```python
from build123d import *

# Parameters (mm, degrees)
F0_R     = 5.3351790251
F1_DEPTH = 10
F2_DEPTH = 10
F3_COUNT = 14
F4_R     = 15.5
F5_DEPTH = 10
F8_DEPTH = 10
F7_R     = 2
F9_DEPTH = 10


# Not quite as in the source:
# - a feature names something its author has since deleted; it is built from what else it names


with BuildPart() as f1:
    # F0 (on Top) → F1 (new body)
    with BuildSketch(Plane.XY):
        Circle(F0_R)
    extrude(amount=F1_DEPTH)



with BuildPart() as f2:
    # F0 (on Top) → F2 (new body)
    with BuildSketch(Plane.XY):
        with BuildLine():
            Line((-21.0813645951, 0), (-15.5169374102, 0))
            Line((-15.5169374102, 0), (-15.5169374102, 2.1929510403))
            add(Edge.make_bspline(
                [(-15.5169374102, 2.1929510403), (-15.7431787684, 2.1963284468), (-16.4584927159, 2.2070069607), (-21.1021855068, 0.9410331304), (-21.0859014535, 0.2050513008), (-21.0813645951, 0)],
                knots=[0, 0, 0, 0, 0.2502118821, 0.7911020914, 1, 1, 1, 1], degree=3))
        make_face()
        Polygon((-15.5169374102, -2.1929510403), (-13.8607590251, -2.1929510403), (-13.8607590251, 2.1929510403), (-15.5169374102, 2.1929510403), (-15.5169374102, 0), align=None)
        with BuildLine():
            add(Edge.make_bspline(
                [(-15.5169374102, -2.1929510403), (-15.7431787684, -2.1963284468), (-16.4584927159, -2.2070069607), (-21.1021855068, -0.9410331304), (-21.0859014535, -0.2050513008), (-21.0813645951, 0)],
                knots=[0, 0, 0, 0, 0.2502118821, 0.7911020914, 1, 1, 1, 1], degree=3))
            Line((-15.5169374102, -2.1929510403), (-15.5169374102, 0))
            Line((-15.5169374102, 0), (-21.0813645951, 0))
        make_face()
    extrude(amount=F2_DEPTH)


with BuildPart() as f3_1:
    # F3: instance of F2
    add(f2.part.rotate(Axis((0, 0, 10), (0, 0, 1)), 1 * 360 / F3_COUNT))


with BuildPart() as f3_2:
    # F3: instance of F2
    add(f2.part.rotate(Axis((0, 0, 10), (0, 0, 1)), 2 * 360 / F3_COUNT))


with BuildPart() as f3_3:
    # F3: instance of F2
    add(f2.part.rotate(Axis((0, 0, 10), (0, 0, 1)), 3 * 360 / F3_COUNT))


with BuildPart() as f3_4:
    # F3: instance of F2
    add(f2.part.rotate(Axis((0, 0, 10), (0, 0, 1)), 4 * 360 / F3_COUNT))


with BuildPart() as f3_5:
    # F3: instance of F2
    add(f2.part.rotate(Axis((0, 0, 10), (0, 0, 1)), 5 * 360 / F3_COUNT))


with BuildPart() as f3_6:
    # F3: instance of F2
    add(f2.part.rotate(Axis((0, 0, 10), (0, 0, 1)), 6 * 360 / F3_COUNT))


with BuildPart() as f3_7:
    # F3: instance of F2
    add(f2.part.rotate(Axis((0, 0, 10), (0, 0, 1)), 7 * 360 / F3_COUNT))


with BuildPart() as f3_8:
    # F3: instance of F2
    add(f2.part.rotate(Axis((0, 0, 10), (0, 0, 1)), 8 * 360 / F3_COUNT))


with BuildPart() as f3_9:
    # F3: instance of F2
    add(f2.part.rotate(Axis((0, 0, 10), (0, 0, 1)), 9 * 360 / F3_COUNT))


with BuildPart() as f3_10:
    # F3: instance of F2
    add(f2.part.rotate(Axis((0, 0, 10), (0, 0, 1)), 10 * 360 / F3_COUNT))


with BuildPart() as f3_11:
    # F3: instance of F2
    add(f2.part.rotate(Axis((0, 0, 10), (0, 0, 1)), 11 * 360 / F3_COUNT))


with BuildPart() as f3_12:
    # F3: instance of F2
    add(f2.part.rotate(Axis((0, 0, 10), (0, 0, 1)), 12 * 360 / F3_COUNT))


with BuildPart() as f3_13:
    # F3: instance of F2
    add(f2.part.rotate(Axis((0, 0, 10), (0, 0, 1)), 13 * 360 / F3_COUNT))


with BuildPart() as f1_1:
    add(f1.part)

    add(f2.part)  # F5 merges F2

    add(f3_1.part)  # F5 merges F3_1

    add(f3_2.part)  # F5 merges F3_2

    add(f3_3.part)  # F5 merges F3_3

    add(f3_4.part)  # F5 merges F3_4

    add(f3_5.part)  # F5 merges F3_5

    add(f3_6.part)  # F5 merges F3_6

    add(f3_7.part)  # F5 merges F3_7

    add(f3_8.part)  # F5 merges F3_8

    add(f3_9.part)  # F5 merges F3_9

    add(f3_10.part)  # F5 merges F3_10

    add(f3_11.part)  # F5 merges F3_11

    add(f3_12.part)  # F5 merges F3_12

    add(f3_13.part)  # F5 merges F3_13
    # F4 (on Top) → F5 (join)
    with BuildSketch(Plane.XY):
        Circle(F4_R)
    extrude(amount=F5_DEPTH)

    # F6 (on face) → F8 (cut, through all)
    with BuildSketch(Plane.XY.offset(10)):
        with BuildLine():
            ThreePointArc((-5.9088465181, -1.041889066), (-5.1961524227, 3), (-2.05212086, 5.6381557247))
            Line((-2.05212086, 5.6381557247), (-4.1564424219, 11.4197316993))
            ThreePointArc((-4.1564424219, 11.4197316993), (-10.5244816627, 6.076312321), (-11.967998967, -2.110281123))
            Line((-11.967998967, -2.110281123), (-5.9088465181, -1.041889066))
        make_face()
        with BuildLine():
            Line((-3.8567256581, -4.5962666587), (-7.8115565451, -9.3094505764))
            ThreePointArc((-7.8115565451, -9.3094505764), (0, -12.1526246421), (7.8115565451, -9.3094505764))
            Line((7.8115565451, -9.3094505764), (3.8567256581, -4.5962666587))
            ThreePointArc((3.8567256581, -4.5962666587), (0, -6), (-3.8567256581, -4.5962666587))
        make_face()
        with BuildLine():
            ThreePointArc((2.05212086, 5.6381557247), (5.1961524227, 3), (5.9088465181, -1.041889066))
            Line((5.9088465181, -1.041889066), (11.967998967, -2.110281123))
            ThreePointArc((11.967998967, -2.110281123), (10.5244816627, 6.076312321), (4.1564424219, 11.4197316993))
            Line((4.1564424219, 11.4197316993), (2.05212086, 5.6381557247))
        make_face()
    extrude(amount=-F8_DEPTH, mode=Mode.SUBTRACT)

    # F7 (on face) → F9 (cut, through all)
    with BuildSketch(Plane.XY.offset(10)):
        Circle(F7_R)
    extrude(amount=-F9_DEPTH, mode=Mode.SUBTRACT)


solid = f1_1.part
```
Source: CAD feature listing. Evaluate the final solid. Frame: model axes, mm. A direction names the side the tool comes from. Round coordinates to 2 decimals unless told otherwise and drop trailing zeros. Write each loop counter-clockwise with the first axis right and the second up, starting at its lowest first coordinate (ties: lowest second). Pieces come first, ordered by that corner, then holes. Notation, with made-up numbers: M -24.5,7 L 7.5,7 A24 ccw 7.5,22 Z; hole C -27,85.25 d8. An arc over 180 degrees is marked long. Answer as a JSON object with one key per item and string values. Group by question number.
(1) Section query A-A on x = 0. Output: boundary loops of the cut face in (y, z).
(2) Section query C-C on z = 5.25. State how many separate pieces and enclosed holes the cut face has, then the cut area to 3 significant figures.
(3) Ray query, line 1 (Y direction, x = 0, z = 7.75); line 2 (X direction, y = 7.5, z = 9.25); line 3 (Y direction, x = -17, z = 1.5). Return the intervals inside material, ascending. Write a range as [from, to].
(4) Section query B-B on x = -7. Output: boundary loops of the cut face in (y, z).
(5) Mould query, pull axis X, two halves, no side actions, for faces 1 (the cylindrical face through (15.1, -3.5, 4.9)), 2 (the flat face through (0, 4, 0)), 3 (the cylindrical face through (12.107, -9.678, 4.93)). Classes: +X half, -X half, draft (parallel to the pull), parting line (faces both ways), or undercut.
(6) First-contact query: pin 1 (3 mm diameter, centred on y = 15.5, z = 7.5, fed in from +X); pin 2 (1.5 mm diameter, centred on y = 14, z = 5, fed in from +X). Flat tips, straight axial feed; report the tip coordinate or a pass-through.
(7) Reachability of faces 4 (the cylindrical face through (5.167, 3.051, 5.07)), 5 (the flat face through (0, 4, 10)), 6 (the cylindrical face through (-15.1, 3.5, 4.9)) from +Z, -Z, +X, -X, +Y, -Y: full face, straight path, thin tool, end or side. Return the list, or none.
Computed values:
{
 "1": {"outline": "M -15.5,0 L -12.15,0 L -12.15,10 L -15.5,10 Z; M -6,0 L -2,0 L -2,10 L -6,10 Z; M 2,0 L 15.5,0 L 15.5,10 L 2,10 Z"},
 "2": {"separate pieces": "1", "enclosed holes": "4", "area": "757 mm^2"},
 "3": {"line 1": "[-15.5, -12.15], [-6, -2], [2, 15.5]", "line 2": "[-18.3, -9.56], [-2.73, 2.73], [9.56, 18.3]", "line 3": "[-9.61, -6.26], [-2, 2], [6.26, 9.61]"},
 "4": {"outline": "M -13.83,0 L -9.93,0 L -9.93,10 L -13.83,10 Z; M -8.34,0 L -1.23,0 L -1.23,10 L -8.34,10 Z; M 9.93,0 L 13.83,0 L 13.83,10 L 9.93,10 Z"},
 "5": {"face 1": "+X half", "face 2": "draft", "face 3": "undercut"},
 "6": {"pin 1": "x = 13.48", "pin 2": "x = 13.25"},
 "7": {"face 4": "+Z, -Z", "face 5": "+Z, +X, -X, +Y, -Y", "face 6": "+Z, -Z, -X"}
}
